from build123d import *

# Parameters (mm, degrees)
F0_W     = 25.5
F0_H     = 20
F1_DEPTH = 5
F2_R     = 2.49999
F3_R     = 1.25
F4_DEPTH = 25
F5_W     = 9.4863112453
F5_H     = 5.25
F5_W_2   = 9.3420613807
F5_H_2   = 5.125
F6_DEPTH = 5.001
F7_R     = 1.5
F8_DEPTH = 25
F9_SIZE  = 2


# Not quite as in the source:
# - a fillet or chamfer is up to 0.001 mm smaller than in the source, because OpenCascade refuses the exact size


with BuildPart() as f1:
    # F0 (on Front) → F1 (new body)
    with BuildSketch(Plane.XZ):
        with Locations((12.75, 10)):
            Rectangle(F0_W, F0_H)
    extrude(amount=F1_DEPTH)

    # F2 (radius 2.5 in the source; OpenCascade refuses exactly that, so slightly less here)
    f2_edges = [f1.edges().sort_by_distance(p)[0] for p in [
        (25.5, -5, 10),
        (25.5, 0, 10),
    ]]
    fillet(f2_edges, radius=F2_R)

    # F3 (on face) → F4 (cut)
    with BuildSketch(Plane.XY.offset(20)):
        with Locations((23, -2.5)):
            Circle(F3_R)
    extrude(amount=-F4_DEPTH, mode=Mode.SUBTRACT)

    # F5 (on face) → F6 (cut, through all)
    with BuildSketch(Plane.XZ.offset(5)):
        with Locations((24.7431556227, 12.5)):
            Rectangle(F5_W, F5_H)
        with Locations((24.6710306904, 2.5625)):
            Rectangle(F5_W_2, F5_H_2)
    extrude(amount=-F6_DEPTH, mode=Mode.SUBTRACT)

    # F7 (on face) → F8 (cut)
    with BuildSketch(Plane.XZ.offset(5)):
        with Locations((14, 10)):
            Circle(F7_R)
        with Locations((6, 15)):
            Circle(F7_R)
        with Locations((6, 5)):
            Circle(F7_R)
    extrude(amount=-F8_DEPTH, mode=Mode.SUBTRACT)

    # F9
    f9_edges = [f1.edges().sort_by_distance(p)[0] for p in [
        (0, -2.5, 20),
        (0, -2.5, 0),
    ]]
    chamfer(f9_edges, length=F9_SIZE)


solid = f1.part
Source: CAD feature listing. Evaluate the final solid. Frame: model axes, mm. A direction names the side the tool comes from. Give positions to 0.01 mm unless a question says otherwise; leave off trailing zeros. Write each loop counter-clockwise with the first axis right and the second up, starting at its lowest first coordinate (ties: lowest second). Pieces come first, ordered by that corner, then holes. Notation, with made-up numbers: M -2.75,72.5 L 2.25,72.5 A26 cw 2.25,89.5 Z; hole C -37,39 d10. An arc over 180 degrees is marked long. Return JSON: item names as keys, results as strings. Group by question number.
1) Pin query (flat end, axial travel): P1, Ø4, axis at x = 14, z = 10, coming from the -Y side; P2, Ø1.5, axis at y = -2, z = 12.5, coming from the +X side. Return the tip coordinate at first contact, or that it passes through.
2) Pull-direction query (X, two-part tool) for faces 1 (the face through (4.89, -2.54, 16.01)), 2 (the face through (14, -2, 20)), 3 (the face through (25, -4, 18)); classes: pulls with the +X half, pulls with the -X half, needs draft (parallel to the pull), parting line crosses it, or undercut.
3) Material intervals for line 1 along Z through (x, y) = (6, -1.2); line 2 along Y through (x, z) = (23, 18.95); line 3 along X through (y, z) = (-2.95, 6), sorted ascending. Write a range as [from, to].
4) Cut plane B-B, the plane x = 14. Output: boundary loops of the cut face in (y, z).
5) Set-up query: faces 4 (the face through (24.155, -2.979, 17.597)), 5 (the face through (20, -3, 3)), 6 (the face through (21, -3, 15.125)). Return all of +Z, -Z, +X, -X, +Y, -Y with unobstructed straight access to the full face (end or side cutting, diameter ignored); none if empty.
6) Cut plane D-D, the plane y = -0.8. Output: boundary loops of the cut face in (x, z) (3 decimals), plus the area to 3 significant figures.
7) Cut plane C-C, the plane x = 6. Output: boundary loops of the cut face in (y, z).
Recorded:
{
 "1": {"P1": "stops at y = -5", "P2": "stops at x = 20"},
 "2": {"face 1": "undercut", "face 2": "needs draft", "face 3": "pulls with the +X half"},
 "3": {"line 1": "z = [0, 3.5], [6.5, 13.5], [16.5, 20]", "line 2": "y = [-5, -3.75], [-1.25, 0]", "line 3": "x = [0, 4.88], [7.12, 21.83], [24.17, 25.46]"},
 "4": {"outline": "M -5,0 L 0,0 L 0,8.5 L -5,8.5 Z; M -5,11.5 L 0,11.5 L 0,20 L -5,20 Z"},
 "5": {"face 4": "+Z, -Z", "face 5": "-Z, +X, +Y, -Y", "face 6": "+X, +Y, -Y"},
 "6": {"outline": "M 0,2 L 2,0 L 20,0 L 20,5.125 L 24.833,5.125 L 24.833,9.875 L 20,9.875 L 20,15.125 L 24.833,15.125 L 24.833,20 L 2,20 L 0,18 Z; hole C 6,5 d3; hole C 6,15 d3; hole C 14,10 d3", "area": "421 mm²"},
 "7": {"outline": "M -5,0 L 0,0 L 0,3.5 L -5,3.5 Z; M -5,6.5 L 0,6.5 L 0,13.5 L -5,13.5 Z; M -5,16.5 L 0,16.5 L 0,20 L -5,20 Z"}
}
